```python
from build123d import *

# Parameters (mm, degrees)
SKETCH_R             = 70
PAD_DEPTH            = 10
SKETCH001_W          = 10
SKETCH001_H          = 20
POCKET_DEPTH         = 5
POLARPATTERN_COUNT   = 12
SKETCH002_R          = 7.5
SKETCH002_R_2        = 5
PAD001_DEPTH         = 20
SKETCH003_R          = 2.5
POCKET001_DEPTH      = 70.001
POCKET001_DEPTH_BACK = -70.001


with BuildPart() as part:
    # Sketch → Pad (new body)
    with BuildSketch(Plane.XY):
        Circle(SKETCH_R)
    extrude(amount=PAD_DEPTH)

    # Sketch001 (on Face2 of Pad) → Pocket (cut)
    with BuildSketch(Plane(origin=(0, 0, 0), x_dir=(1, 0, 0), z_dir=(0, 0, -1))):
        with Locations((0, 40)):
            Rectangle(SKETCH001_W, SKETCH001_H)
    pocket = extrude(amount=-POCKET_DEPTH, mode=Mode.SUBTRACT)

    # PolarPattern: Pocket ×12 about axis
    polarpattern_axis = Axis((0, 0, 0), (0, 0, -1))
    for i in range(1, POLARPATTERN_COUNT):
        add(pocket.rotate(polarpattern_axis, i * 360 / POLARPATTERN_COUNT), mode=Mode.SUBTRACT)

    # Sketch002 (on Face3 of PolarPattern) → Pad001 (join)
    with BuildSketch(Plane.XY.offset(10)):
        Circle(SKETCH002_R)
        Circle(SKETCH002_R_2, mode=Mode.SUBTRACT)
    extrude(amount=PAD001_DEPTH)

    # Sketch003 → Pocket001 (cut, two sides)
    with BuildSketch(Plane.YZ) as pocket001_sk:
        with Locations((0, 20)):
            Circle(SKETCH003_R)
    extrude(amount=-POCKET001_DEPTH, mode=Mode.SUBTRACT)
    extrude(pocket001_sk.sketch, amount=-POCKET001_DEPTH_BACK, mode=Mode.SUBTRACT)


solid = part.part
```
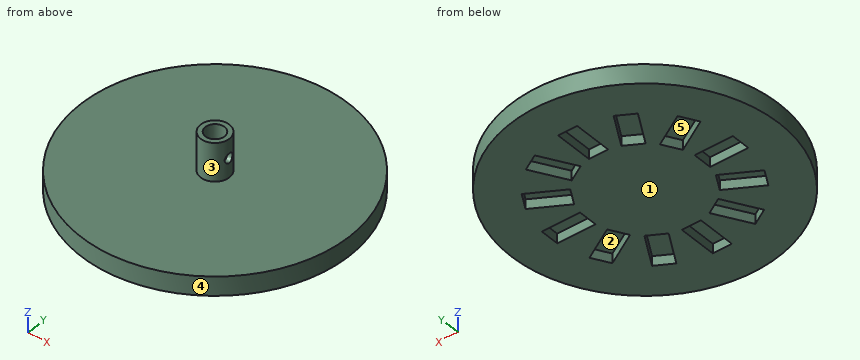
Check sheet for the modelled part. Datum: model origin and axes. Units: mm. Face numbers are marked on the shaded views. A direction names the side the tool comes from. Give positions to 0.01 mm unless a question says otherwise; leave off trailing zeros. Order: outer loops, then holes, each group sorted by start corner. A loop starts at its lowest first (then second) coordinate and runs counter-clockwise, first axis right, second up. Notation, with made-up numbers: (-20.5, 18.5) -> (6.5, 18.5) arc R24 ccw to (6.5, 30.5) -> close; hole circle Ø4 at (78.5, 7). An arc over 180 degrees is marked (long way). Use CSV: the item, a comma, the result in double quotes. Start each with the question number.
1) Set-up check for the marked faces 4 and 5: record each of +Z, -Z, +X, -X, +Y, -Y from which the full face is reachable in a straight line by a thin tool's end or side.
2) Sectioned sample at B-B, the plane x = 0. Record the boundary of the cut face in (y, z).
3) Sectioned sample at D-D, the plane y = 34. Record the boundary of the cut face in (x, z).
4) Sectioned sample at C-C, the plane z = 20. Record the boundary of the cut face in (x, y), plus the area to 3 significant figures.
5) Sectioned sample at A-A, the plane y = 0. Record the boundary of the cut face in (x, z).
6) Material ranges on line 1 (X direction, y = 0, z = 15.25); line 2 (X direction, y = -33.5, z = 2.5); line 3 (Z direction, x = 5.75, y = 0), recorded low to high. Write a range as from..to.
7) Go/stop test with flat-tipped pins: P1, Ø9, axis at x = 0, y = 0, coming from the +Z side; P2, Ø5.5, axis at x = 37, y = 19.5, coming from the -Z side; P3, Ø5.5, axis at x = 41, z = 1.5, coming from the -Y side; P4, Ø10, axis at y = -16.5, z = 27, coming from the +X side. Record where each tip stops, or that it passes through.
8) Mould release check, pull along X, two halves, no side actions. Record for the marked faces 1, 2 and 3: released by +X, released by -X, zero draft, split by the parting line, or undercut.
Recorded:
1,face 4,"+Z, -Z"
1,face 5,"-Z"
2,outline,"(-70, 0) -> (-50, 0) -> (-50, 5) -> (-30, 5) -> (-30, 0) -> (30, 0) -> (30, 5) -> (50, 5) -> (50, 0) -> (70, 0) -> (70, 10) -> (7.5, 10) -> (7.5, 30) -> (5, 30) -> (5, 10) -> (-5, 10) -> (-5, 30) -> (-7.5, 30) -> (-7.5, 10) -> (-70, 10) -> close"
3,outline,"(-61.19, 0) -> (-25.4, 0) -> (-25.4, 5) -> (-13.86, 5) -> (-13.86, 0) -> (-5, 0) -> (-5, 5) -> (5, 5) -> (5, 0) -> (13.86, 0) -> (13.86, 5) -> (25.4, 5) -> (25.4, 0) -> (61.19, 0) -> (61.19, 10) -> (-61.19, 10) -> close"
4,outline,"(-7.07, -2.5) arc R7.5 ccw to (7.07, -2.5) -> (4.33, -2.5) arc R5 cw to (-4.33, -2.5) -> close; (-7.07, 2.5) -> (-4.33, 2.5) arc R5 cw to (4.33, 2.5) -> (7.07, 2.5) arc R7.5 ccw to start"
4,area,"72.4 mm2"
5,outline,"(-70, 0) -> (-50, 0) -> (-50, 5) -> (-30, 5) -> (-30, 0) -> (30, 0) -> (30, 5) -> (50, 5) -> (50, 0) -> (70, 0) -> (70, 10) -> (7.5, 10) -> (7.5, 17.5) -> (5, 17.5) -> (5, 10) -> (-5, 10) -> (-5, 17.5) -> (-7.5, 17.5) -> (-7.5, 10) -> (-70, 10) -> close; (-7.5, 22.5) -> (-5, 22.5) -> (-5, 30) -> (-7.5, 30) -> close; (5, 22.5) -> (7.5, 22.5) -> (7.5, 30) -> (5, 30) -> close"
6,line 1,"-7.5..-5, 5..7.5"
6,line 2,"-61.46..-25.11, -13.57..-5, 5..13.57, 25.11..61.46"
6,line 3,"0..17.5, 22.5..30"
7,P1,"z = 10"
7,P2,"z = 5"
7,P3,"y = -58.63"
7,P4,"through"
8,face 1,"zero draft"
8,face 2,"undercut"
8,face 3,"split by the parting line"
